```python
from build123d import *

# Parameters (mm, degrees)
F0_R         = 101
F0_R_2       = 4
F1_DEPTH     = 5
F2_R         = 15.5
F2_R_2       = 3
F1_FACE1_R   = 101
F1_FACE1_R_2 = 4
F3_DEPTH     = 10.001
F5_R         = 55.5
F6_DEPTH     = 1.5
F7_R         = 55.5
F4_DEPTH     = 2.5


with BuildPart() as f1:
    # F0 (on Front) → F1 (new body, symmetric)
    with BuildSketch(Plane.XZ):
        Circle(F0_R)
        Circle(F0_R_2, mode=Mode.SUBTRACT)
    extrude(amount=F1_DEPTH, both=True)

    # F2 (on face) + F1_face1 (on face) → F3 (cut, through all)
    with BuildSketch(Plane.XZ.offset(5)):
        with Locations((-55.5078823231, -55.5078823231)):
            Circle(F2_R)
        with Locations((-78.5, 0)):
            Circle(F2_R)
        with Locations((-55.5078823231, 55.5078823231)):
            Circle(F2_R)
        with Locations((0, 78.5)):
            Circle(F2_R)
        with Locations((55.5078823231, 55.5078823231)):
            Circle(F2_R)
        with Locations((78.5, 0)):
            Circle(F2_R)
        with Locations((55.5078823231, -55.5078823231)):
            Circle(F2_R)
        with Locations((0, -78.5)):
            Circle(F2_R)
        with Locations((-20, 20)):
            Circle(F2_R_2)
        with Locations((20, 20)):
            Circle(F2_R_2)
        with Locations((20, -20)):
            Circle(F2_R_2)
        with Locations((-20, -20)):
            Circle(F2_R_2)
    with BuildSketch(Plane(origin=(0, 5, 0), x_dir=(1, 0, 0), z_dir=(0, 1, 0))):
        Circle(F1_FACE1_R)
        Circle(F1_FACE1_R_2, mode=Mode.SUBTRACT)
    extrude(amount=-F3_DEPTH, dir=(0, -1, 0), mode=Mode.SUBTRACT)

    # F5 (on face) → F6 (cut, symmetric)
    with BuildSketch(Plane.XZ.offset(5)):
        Circle(F5_R)
    extrude(amount=F6_DEPTH, both=True, mode=Mode.SUBTRACT)

    # F7 (on face) → F4 (cut, symmetric)
    with BuildSketch(Plane(origin=(0, 5, 0), x_dir=(-1, 0, 0), z_dir=(0, 1, 0))):
        Circle(F7_R)
    extrude(amount=F4_DEPTH, both=True, mode=Mode.SUBTRACT)


solid = f1.part
```
The listing builds one solid part. Answer for the finished solid, in the listing's coordinates (mm). A direction names the side the tool comes from. Coordinates: 2 decimals unless noted, no trailing zeros. Write each loop counter-clockwise with the first axis right and the second up, starting at its lowest first coordinate (ties: lowest second). Pieces come first, ordered by that corner, then holes. Notation, with made-up numbers: (75.5, -24) -> (119.5, -24) arc R29 cw to (119.5, -4) -> close; hole circle Ø11 at (18, 26.25). An arc over 180 degrees is marked (long way). Write each question's results on one line, items separated by ' | '. Start each with the question number.
1) A cutting plane is placed at A-A (x = 68.5). Determine the outline of the cut face in (y, z), then the cut area to 3 significant figures.
2) A cutting plane is placed at B-B (z = -20). Determine the outline of the cut face in (x, y).
3) A cutting plane is placed at C-C (x = -84). Determine the outline of the cut face in (y, z), then the cut area to 3 significant figures.
4) Flat-ended cylindrical pins translate along their axes: pin 1 Ø2 at (y, z) = (1, -23) entering from +X; pin 2 Ø4 at (x, z) = (-22.5, 10) entering from -Y; pin 3 Ø1 at (x, y) = (22.5, 1.5) entering from +Z. Find the tip coordinate at first contact, or state that the pin passes through.
5) Straight lines are drawn through the part: probe 1 along Z at (x, y) = (10.5, -2.75); probe 2 along X at (y, z) = (-2, -65.5); probe 3 along Z at (x, y) = (-12, -4). For each, find the intervals that lie inside material, in ascending order.
6) For a pull along Z with two mould halves and no side action, classify faces 4 (the flat face through (43, -5, -43)), 5 (the cylindrical face through (-21.89, -0.07, -98.6)), 6 (the cylindrical face through (-93.985, -0.07, 0.682)) as +Z half, -Z half, draft (parallel to the pull), parting line (faces both ways), or undercut.
7) A cutting plane is placed at D-D (x = -20). Determine the outline of the cut face in (y, z), then the cut area to 3 significant figures.
8) A tool of negligible diameter and unlimited length cuts with its end or side. For faces 1 (the flat face through (-1, -3.5, -12)), 2 (the flat face through (1, 2.5, -12)), 3 (the cylindrical face through (63.015, -0.07, 0.682)), from which of +Z, -Z, +X, -X, +Y, -Y can it reach the whole face along a straight path? Write none if from no direction.
Values follow:
1) outline: (-5, -74.22) -> (5, -74.22) -> (5, -63.96) -> (-5, -63.96) -> close; (-5, -47.05) -> (5, -47.05) -> (5, -11.84) -> (-5, -11.84) -> close; (-5, 11.84) -> (5, 11.84) -> (5, 47.05) -> (-5, 47.05) -> close; (-5, 63.96) -> (5, 63.96) -> (5, 74.22) -> (-5, 74.22) -> close | area: 909 mm²
2) outline: (-99, -5) -> (-51.77, -5) -> (-51.77, -3.5) -> (-23, -3.5) -> (-23, 2.5) -> (-51.77, 2.5) -> (-51.77, 5) -> (-99, 5) -> close; (-17, -3.5) -> (17, -3.5) -> (17, 2.5) -> (-17, 2.5) -> close; (23, -3.5) -> (51.77, -3.5) -> (51.77, -5) -> (99, -5) -> (99, 5) -> (51.77, 5) -> (51.77, 2.5) -> (23, 2.5) -> close
3) outline: (-5, -56.08) -> (5, -56.08) -> (5, -14.49) -> (-5, -14.49) -> close; (-5, 14.49) -> (5, 14.49) -> (5, 56.08) -> (-5, 56.08) -> close | area: 832 mm²
4) pin 1: x = 98.57 | pin 2: y = -3.5 | pin 3: z = 98.57
5) probe 1: -100.45 to -89.9, -67.1 to 67.1, 89.9 to 100.45 | probe 2: -76.88 to -67.36, -43.66 to -8.44, 8.44 to 43.66, 67.36 to 76.88 | probe 3: -100.28 to -88.31, -68.69 to -54.19, 54.19 to 68.69, 88.31 to 100.28
6) face 4: draft | face 5: parting line | face 6: undercut
7) outline: (-5, -99) -> (5, -99) -> (5, -51.77) -> (2.5, -51.77) -> (2.5, -23) -> (-3.5, -23) -> (-3.5, -51.77) -> (-5, -51.77) -> close; (-5, 51.77) -> (-3.5, 51.77) -> (-3.5, 23) -> (2.5, 23) -> (2.5, 51.77) -> (5, 51.77) -> (5, 99) -> (-5, 99) -> close; (-3.5, -17) -> (2.5, -17) -> (2.5, 17) -> (-3.5, 17) -> close | area: 1,490 mm²
8) face 1: -Y | face 2: +Y | face 3: +Y, -Y
